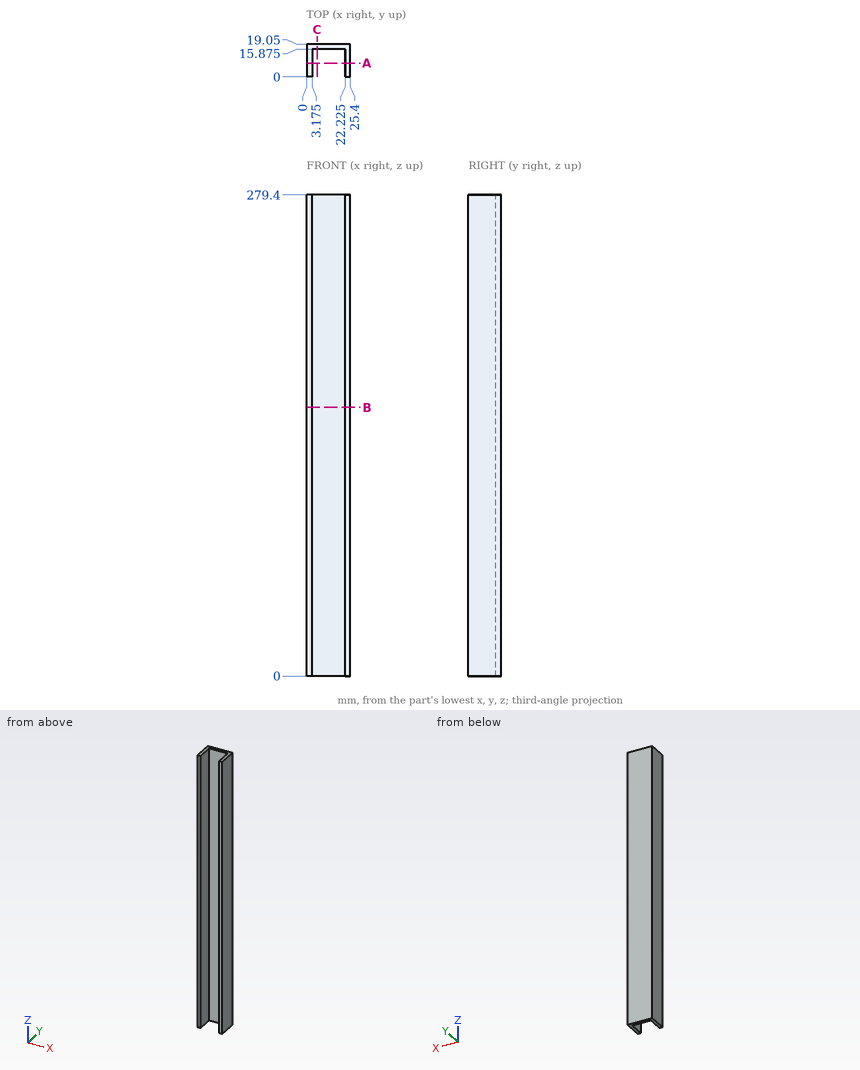
Can you work these out from the drawing? Everything is in mm from the part's minimum corner. Coordinates: 2 decimals unless noted, no trailing zeros. Loops run counter-clockwise (first coordinate to the right, second up) from the corner with the lowest first, then second, coordinate; pieces in that order, holes last.
1) I need wall thicknesses on probe 1 along X at (y, z) = (2.5, 253) (3 decimals); probe 2 along Y at (x, z) = (12.75, 143) (3 decimals). Which ranges of each line are inside material? Lowest first, please.
2) Imagine slicing it at A-A on y = 8. List the corners of the cut face in (x, z) for me (3 decimals).
3) Imagine slicing it at C-C on x = 6. List the corners of the cut face in (y, z) for me (3 decimals), plus the area to 3 significant figures.
4) For pin 1 (1 mm diameter, centred on x = 18.5, z = 175.5, fed in from -Y) (3 decimals), with a flat end and sliding along its axis, tell me the tip position at first contact or that it passes through.
5) Imagine slicing it at B-B on z = 156. List the corners of the cut face in (x, y) for me (3 decimals).
Completed:
1. probe 1: x = 0 to 3.175, 22.225 to 25.4
1. probe 2: y = 15.875 to 19.05
2. outline: (0, 0) - (3.175, 0) - (3.175, 279.4) - (0, 279.4) - close; (22.225, 0) - (25.4, 0) - (25.4, 279.4) - (22.225, 279.4) - close
3. outline: (15.875, 0) - (19.05, 0) - (19.05, 279.4) - (15.875, 279.4) - close
3. area: 887 mm2
4. pin 1: stops at y = 15.875
5. outline: (0, 0) - (3.175, 0) - (3.175, 15.875) - (22.225, 15.875) - (22.225, 0) - (25.4, 0) - (25.4, 19.05) - (0, 19.05) - close
